Design review of the part shown in the three views and the two pictorial views. Dimensions are in mm from the part's minimum x, y and z. A direction names the side the tool comes from. Coordinates: 2 decimals unless noted, no trailing zeros. Loops run counter-clockwise (first coordinate to the right, second up) from the corner with the lowest first, then second, coordinate; pieces in that order, holes last. Notation, with made-up numbers: (-13.5, 66) -> (-4.5, 66) arc R18 ccw to (-4.5, 99) -> close; hole circle Ø5 at (-34.75, 62.25). An arc over 180 degrees is marked (long way). Use CSV: the item, a comma, the result in double quotes.
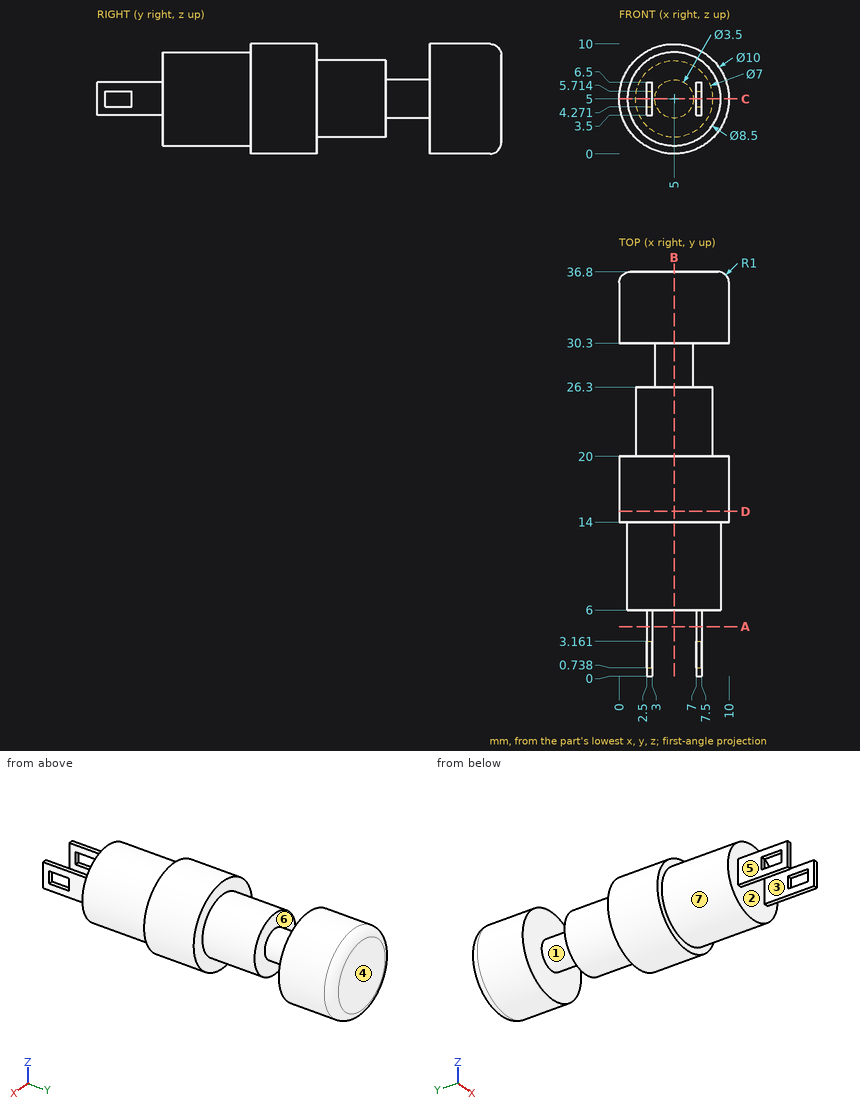
Item 1: Clearance check with flat-ended pins moving along their axes: pin 1 (2.5 mm diameter, centred on y = 2.5, z = 4.5, fed in from -X); pin 2 (3 mm diameter, centred on y = 30.5, z = 1.5, fed in from -X); pin 3 (0.6 mm diameter, centred on x = 2.5, y = 1.5, fed in from +Z). State where each tip first meets the part, or that it passes through.
Checked values:
pin 1,"x = 2.5"
pin 2,"x = 0.42"
pin 3,"z = 6.5"
Item 2: Draft analysis for pull direction X (two halves, no side actions). For the marked faces 1, 2, 3 and 4, state which applies: pulls with the +X half, pulls with the -X half, needs draft (parallel to the pull), parting line crosses it, or undercut.
Checked values:
face 1,"parting line crosses it"
face 2,"undercut"
face 3,"undercut"
face 4,"needs draft"
Item 3: Add section A-A (y = 4.5). Give the boundary of the cut face in (x, z).
Checked values:
outline,"(2.5, 3.5) -> (3, 3.5) -> (3, 6.5) -> (2.5, 6.5) -> close; (7, 3.5) -> (7.5, 3.5) -> (7.5, 6.5) -> (7, 6.5) -> close"
Item 4: Machinability: for the marked faces 5, 6 and 7, which of the approach directions +Z, -Z, +X, -X, +Y, -Y give a long, thin tool a straight path to every point of the face, cutting with its end or side? Answer none if there is none.
Checked values:
face 5,"+Z, -Z, -X, -Y"
face 6,"none"
face 7,"-Y"
Item 5: To check wall thickness, follow line 1 along Y through (x, z) = (5, 7); line 2 along Y through (x, z) = (8, 7.25); line 3 along Y through (x, z) = (5.75, 5.75). State the ranges of each line that lie inside material, in increasing order.
Checked values:
line 1,"6 to 26.3, 30.3 to 36.8"
line 2,"6 to 20, 30.3 to 36.8"
line 3,"6 to 36.8"
Item 6: Add section B-B (x = 5). Give the boundary of the cut face in (y, z), then the cut area to 3 significant figures.
Checked values:
outline,"(6, 0.75) -> (14, 0.75) -> (14, 0) -> (20, 0) -> (20, 1.5) -> (26.3, 1.5) -> (26.3, 3.25) -> (30.3, 3.25) -> (30.3, 0) -> (35.8, 0) arc R1 ccw to (36.8, 1) -> (36.8, 9) arc R1 ccw to (35.8, 10) -> (30.3, 10) -> (30.3, 6.75) -> (26.3, 6.75) -> (26.3, 8.5) -> (20, 8.5) -> (20, 10) -> (14, 10) -> (14, 9.25) -> (6, 9.25) -> close"
area,"251 mm^2"
Item 7: Add section D-D (y = 15). Give the boundary of the cut face in (x, z).
Checked values:
outline,"circle Ø10 at (5, 5)"
Item 8: Add section C-C (z = 5). State how many separate pieces and enclosed holes the cut face has, then the cut area to 3 significant figures.
Checked values:
separate pieces,"3"
enclosed holes,"0"
area,"254 mm^2"
